from build123d import *

# Parameters (mm, degrees)
SKETCH1_W           = 25.4
SKETCH1_H           = 25.4
BOSS_EXTRUDE1_DEPTH = 25.4
SHELL1_T            = -2
SKETCH2_R           = 0.5
CUT_EXTRUDE1_DEPTH  = 6.4
SKETCH3_R           = 0.5
CUT_EXTRUDE2_DEPTH  = 6.4
SHELL2_START        = 1.5
SHELL2_OUTLINE_W    = 0.5
SHELL2_OUTLINE_H    = 22.4
SHELL2_DEPTH        = 22.4


# Read off the part's stored shape, not the designer's step: Shell2
with BuildPart() as part:
    # Sketch1 → Boss-Extrude1 (new body)
    with BuildSketch(Plane(origin=(0, 0, 0), x_dir=(1, 0, 0), z_dir=(0, 1, 0))):
        Rectangle(SKETCH1_W, SKETCH1_H)
    extrude(amount=BOSS_EXTRUDE1_DEPTH)

    # Shell1
    shell1_openings = [part.faces().sort_by_distance(p)[0] for p in [
        (0, 25.4, 0),
    ]]
    offset(amount=SHELL1_T, openings=shell1_openings, kind=Kind.INTERSECTION)

    # Sketch2 → Cut-Extrude1 (cut)
    with BuildSketch(Plane(origin=(12.7, 0, 0), x_dir=(0, 0, -1), z_dir=(1, 0, 0))):
        with Locations((0, 9.984928122)):
            Circle(SKETCH2_R)
    extrude(amount=-CUT_EXTRUDE1_DEPTH, mode=Mode.SUBTRACT)

    # Sketch3 → Cut-Extrude2 (cut)
    with BuildSketch(Plane(origin=(12.7, 0, 0), x_dir=(0, 0, -1), z_dir=(1, 0, 0))):
        with Locations((0, 16.669636536)):
            Circle(SKETCH3_R)
    extrude(amount=-CUT_EXTRUDE2_DEPTH, mode=Mode.SUBTRACT)

    # Shell2 outline → Shell2 (cut)
    with BuildSketch(Plane(origin=(0, 0, 0), x_dir=(1, 0, 0), z_dir=(0, 1, 0)).offset(SHELL2_START)):
        with Locations((-12.45, 0)):
            Rectangle(SHELL2_OUTLINE_W, SHELL2_OUTLINE_H)
    extrude(amount=SHELL2_DEPTH, mode=Mode.SUBTRACT)


solid = part.part
Can you work these out from the model? Positions are in its coordinate system, mm. A direction names the side the tool comes from. Round coordinates to 2 decimals unless told otherwise and drop trailing zeros. Order: outer loops, then holes, each group sorted by start corner. A loop starts at its lowest first (then second) coordinate and runs counter-clockwise, first axis right, second up. Notation, with made-up numbers: (-7, -26.5) -> (48, -26.5) arc R23 cw to (48, 12.5) -> close; hole circle Ø3 at (66, 74). An arc over 180 degrees is marked (long way). Write each question's results on one line, items separated by ' | '. Start each with the question number.
Item 1: If we section it at B-B, the plane y = 2.5: Write out the boundary of the cut face in (x, z), then the cut area to 3 significant figures.
Item 2: Thinking about a two-plate mould opening in Z: for faces 1 (the flat face through (0, 13, -12.7)), 2 (the flat face through (0, 2, 0)), 3 (the flat face through (0, 14, -10.7)), 4 (the flat face through (0, 13, 12.7)), which applies, +Z half, -Z half, draft (parallel to the pull), parting line (faces both ways), or undercut?
Item 3: If we section it at C-C, the plane x = 0: Write out the boundary of the cut face in (y, z), then the cut area to 3 significant figures.
Item 4: Please list where these lines run through material, in increasing order: L1, parallel to Z at x = 3.5, y = 16.25; L2, parallel to X at y = 10.75, z = 3.75; L3, parallel to Y at x = 11.5, z = 0.
Item 5: Will these pins go through, and if not, where does the flat tip stop? pin 1 (11 mm diameter, centred on y = 10, z = -2, fed in from -X); pin 2 (6.5 mm diameter, centred on x = -4, z = 2.5, fed in from +Y).
Item 6: If we section it at A-A, the plane z = 0: Write out the boundary of the cut face in (x, y), then the cut area to 3 significant figures.
Item 7: Which directions (+Z, -Z, +X, -X, +Y, -Y) give clear straight access to the entire face, cutting with the end or side of a thin tool? Please do faces 5 (the cylindrical face through (11.71, 10.48, 0.07)), 6 (the flat face through (-10.7, 14, 0)), 7 (the flat face through (-12.2, 13, 0)).
Results:
1) outline: (-12.7, -12.7) -> (12.7, -12.7) -> (12.7, 12.7) -> (-12.7, 12.7) -> (-12.7, 11.2) -> (-12.2, 11.2) -> (-12.2, -11.2) -> (-12.7, -11.2) -> close; hole (-10.7, -10.7) -> (10.7, -10.7) -> (10.7, 10.7) -> (-10.7, 10.7) -> close | area: 176 mm2
2) face 1: -Z half | face 2: undercut | face 3: undercut | face 4: +Z half
3) outline: (0, -12.7) -> (25.4, -12.7) -> (25.4, -10.7) -> (2, -10.7) -> (2, 10.7) -> (25.4, 10.7) -> (25.4, 12.7) -> (0, 12.7) -> close | area: 144 mm2
4) L1: z = -12.7 to -10.7, 10.7 to 12.7 | L2: x = -12.2 to -10.7, 10.7 to 12.7 | L3: y = 0 to 9.48, 10.48 to 16.17, 17.17 to 25.4
5) pin 1: stops at x = -12.2 | pin 2: stops at y = 2
6) outline: (-12.7, 0) -> (12.7, 0) -> (12.7, 9.48) -> (10.7, 9.48) -> (10.7, 2) -> (-10.7, 2) -> (-10.7, 25.4) -> (-12.7, 25.4) -> (-12.7, 23.9) -> (-12.2, 23.9) -> (-12.2, 1.5) -> (-12.7, 1.5) -> close; (10.7, 10.48) -> (12.7, 10.48) -> (12.7, 16.17) -> (10.7, 16.17) -> close; (10.7, 17.17) -> (12.7, 17.17) -> (12.7, 25.4) -> (10.7, 25.4) -> close | area: 129 mm2
7) face 5: +X | face 6: +Y | face 7: -X
